Autodesk Inventor part; units mm, degrees
ref_plane "YZ Plane" through (0, 0, 0) normal (1, 0, 0) x (0, 1, 0)
ref_plane "XZ Plane" through (0, 0, 0) normal (0, 1, 0) x (-1, 0, 0)
ref_plane "XY Plane" through (0, 0, 0) normal (0, 0, 1) x (1, 0, 0)
sketch "Sketch1" plane through (0, 0, 0) normal (0, 1, 0) x (-1, 0, 0)
  circle A0 centre (0, 0) radius 5
  circle A1 centre (0.7051, 2.7925) radius 2
  circle A2 centre (-1.6909, -2.1323) radius 2
  circle A3 centre (2.4362, -1.3202) radius 2
  circle A4 centre (-2.8575, 2.0067) radius 1.35
  circle A5 centre (3.5172, 1.7971) radius 0.75
  circle A6 centre (0.9671, -3.8612) radius 0.75
  circle A7 centre (-3.984, -0.1323) radius 0.75
  point P0 (2.4362, -7.492)
  point P1 (2.4362, -7.492)
  dimension "d0" = 10
  dimension "d1" = 4
  dimension "d2" = 4
  dimension "d3" = 4
  dimension "d5" = 2.7
  dimension "d6" = 1.5
  dimension "d7" = 1.5
  dimension "d8" = 1.5
extrude "Extrusion1" add sketch "Sketch1" along normal blind 130
sketch "Sketch2" plane through (0, 0, 0) normal (0, -1, 0) x (1, 0, 0)
  point P0 (0, 0)
sketch "Sketch3" plane through (0, 0, 0) normal (0, -1, 0) x (1, 0, 0)
  point P0 (0, 0)
properties part number "outer casing"
Part model, mm, in its own coordinate system. Coordinates: 2 decimals unless noted, no trailing zeros. Loops run counter-clockwise (first coordinate to the right, second up) from the corner with the lowest first, then second, coordinate; pieces in that order, holes last. Notation, with made-up numbers: (60.5, 85.25) -> (84.5, 85.25) arc R22 ccw to (84.5, 121.25) -> close; hole circle Ø4 at (36, 76.25). An arc over 180 degrees is marked (long way). Use a Markdown table: item, result. Add a question column.
Item 1: Pull direction Z, two halves, no side cores. Call faces 1 (the cylindrical face through (3.033, 64.09, 0.668)), 2 (the cylindrical face through (1.08, 64.09, 4.88)), 3 (the flat face through (0, 130, 0)): +Z half, -Z half, draft (parallel to the pull), parting line (faces both ways), or undercut.
Item 2: Flat gauge pins, fed straight in: P1, Ø5, axis at x = -3.5, z = -1.5, coming from the +Y side; P2, Ø1, axis at x = -3.5, y = 60.5, coming from the +Z side; P3, Ø3, axis at x = -3.5, y = 74.5, coming from the -Z side; P4, Ø1, axis at y = 72.5, z = 3.5, coming from the -X side. Where does each tip first touch, or does it go through?
Item 3: Band-saw the part on A-A on y = 10. Write the cut outline in (x, z).
Item 4: Probe probe 1 along X at (y, z) = (9, -3.5); probe 2 along X at (y, z) = (32, 0.5); probe 3 along Z at (x, y) = (0.25, 73). List the from-to ranges inside material, lowest first.
Geometry says:
| question | item | result |
|---|---|---|
| 1 | face 1 | undercut |
| 1 | face 2 | parting line |
| 1 | face 3 | draft |
| 2 | P1 | y = 130 |
| 2 | P2 | z = 4 |
| 2 | P3 | z = -4.58 |
| 2 | P4 | x = -4 |
| 3 | outline | circle Ø10 at (0, 0); hole circle Ø4 at (-2.44, -1.32); hole circle Ø1.5 at (-3.52, 1.8); hole circle Ø4 at (-0.71, 2.79); hole circle Ø1.5 at (-0.97, -3.86); hole circle Ø4 at (1.69, -2.13); hole circle Ø2.7 at (2.86, 2.01); hole circle Ø1.5 at (3.98, -0.13) |
| 4 | probe 1 | -3.57 to -1.62, -0.31 to 0.23, 3.15 to 3.57 |
| 4 | probe 2 | -4.97 to -3.26, -1.61 to 3.58, 4.39 to 4.97 |
| 4 | probe 3 | -4.99 to -3.52, -0.75 to 1.04, 4.55 to 4.99 |
